from build123d import *

# Parameters (mm, degrees)
SKETCH_W               = 8.5
SKETCH_H               = 8.5
PAD_DEPTH              = 113.5
SKETCH001_W            = 10
SKETCH001_H            = 10
POCKET_DEPTH           = 2.5
LINEARPATTERN_COUNT    = 4
LINEARPATTERN_PITCH    = 20
SKETCH002_W            = 10
SKETCH002_H            = 10
POCKET001_DEPTH        = 2.5
LINEARPATTERN001_COUNT = 4
LINEARPATTERN001_PITCH = 20
FILLET_R               = 1
SKETCH003_R            = 1.25
POCKET002_DEPTH        = 6.001
LINEARPATTERN002_COUNT = 4
LINEARPATTERN002_PITCH = 20
SKETCH004_R            = 1.25
POCKET003_DEPTH        = 6.001
LINEARPATTERN003_COUNT = 4
LINEARPATTERN003_PITCH = 20


with BuildPart() as part:
    # Sketch → Pad (new body)
    with BuildSketch(Plane.XY):
        with Locations((4.25, 4.25)):
            Rectangle(SKETCH_W, SKETCH_H)
    extrude(amount=PAD_DEPTH)

    # Sketch001 → Pocket (cut)
    with BuildSketch(Plane.XZ):
        with Locations((4.410969, 21)):
            Rectangle(SKETCH001_W, SKETCH001_H)
    pocket = extrude(amount=-POCKET_DEPTH, mode=Mode.SUBTRACT)

    # LinearPattern: Pocket ×4
    with Locations(*[(0, 0, i * LINEARPATTERN_PITCH) for i in range(1, LINEARPATTERN_COUNT)]):
        add(pocket, mode=Mode.SUBTRACT)

    # Sketch002 → Pocket001 (cut)
    with BuildSketch(Plane(origin=(0, 0, 0), x_dir=(0, -1, 0), z_dir=(-1, 0, 0))):
        with Locations((-4.326825, 31)):
            Rectangle(SKETCH002_W, SKETCH002_H)
    pocket001 = extrude(amount=-POCKET001_DEPTH, mode=Mode.SUBTRACT)

    # LinearPattern001: Pocket001 ×4
    with Locations(*[(0, 0, i * LINEARPATTERN001_PITCH) for i in range(1, LINEARPATTERN001_COUNT)]):
        add(pocket001, mode=Mode.SUBTRACT)

    # Fillet
    fillet_edges = [part.edges().sort_by_distance(p)[0] for p in [
        (8.5, 8.5, 56.75),
    ]]
    fillet(fillet_edges, radius=FILLET_R)

    # Sketch003 → Pocket002 (cut, through all)
    with BuildSketch(Plane.XZ.offset(-2.5)):
        with Locations((5.25, 21)):
            Circle(SKETCH003_R)
    pocket002 = extrude(amount=-POCKET002_DEPTH, mode=Mode.SUBTRACT)

    # LinearPattern002: Pocket002 ×4
    with Locations(*[(0, 0, i * LINEARPATTERN002_PITCH) for i in range(1, LINEARPATTERN002_COUNT)]):
        add(pocket002, mode=Mode.SUBTRACT)

    # Sketch004 → Pocket003 (cut, through all)
    with BuildSketch(Plane(origin=(2.5, 0, 0), x_dir=(0, -1, 0), z_dir=(-1, 0, 0))):
        with Locations((-5.25, 31)):
            Circle(SKETCH004_R)
    pocket003 = extrude(amount=-POCKET003_DEPTH, mode=Mode.SUBTRACT)

    # LinearPattern003: Pocket003 ×4
    with Locations(*[(0, 0, i * LINEARPATTERN003_PITCH) for i in range(1, LINEARPATTERN003_COUNT)]):
        add(pocket003, mode=Mode.SUBTRACT)


solid = part.part
Build history of the part. All positions in model axes, mm. A direction names the side the tool comes from. Coordinates: 2 decimals unless noted, no trailing zeros. Write each loop counter-clockwise with the first axis right and the second up, starting at its lowest first coordinate (ties: lowest second). Pieces come first, ordered by that corner, then holes. Notation, with made-up numbers: (80.5, 18) -> (84.5, 18) arc R32 cw to (84.5, 52) -> close; hole circle Ø6 at (87.25, 72). An arc over 180 degrees is marked (long way). Use CSV: the item, a comma, the result in double quotes. Start each with the question number.
Q1. 3-axis set-ups, long thin cutter, end or side, ignore diameter. For faces 3 (the flat face through (2.5, 3, 91)), 4 (the cylindrical face through (5.46, 5.41, 52.24)), 5 (the flat face through (5, 1, 76)): which of +Z, -Z, +X, -X, +Y, -Y reach the whole face in a straight line?
Q2. Cut at B-B, the plane y = 5. State how many separate pieces and enclosed holes the cut face has, then the cut area to 3 significant figures.
Q3. Cut at C-C, the plane z = 44.5. List the corners of the cut face in (x, y), then the cut area to 3 significant figures.
Q4. Flat gauge pins, fed straight in: pin 1 Ø1.2 at (x, y) = (1.5, 5) entering from -Z; pin 2 Ø4 at (y, z) = (5.5, 29) entering from -X; pin 3 Ø2.5 at (x, z) = (4, 62) entering from -Y; pin 4 Ø1.5 at (x, z) = (5.25, 81) entering from +Y. Where does each tip first touch, or does it go through?
Q5. Cut at A-A, the plane z = 21. List the corners of the cut face in (x, y).
Q6. Pull direction Z, two halves, no side cores. Call faces 1 (the flat face through (4, 8.5, 56)), 2 (the flat face through (1, 6, 26)): released by +Z, released by -Z, zero draft, split by the parting line, or undercut.
Q7. Drill centre lines: probe 1 along Z at (x, y) = (5, 1); probe 2 along Z at (x, y) = (1, 7.25); probe 3 along Y at (x, z) = (6, 18). Where is each one in solid material? Low to high.
Checked values:
1,face 3,"-X, +Y, -Y"
1,face 4,"+X, -X"
1,face 5,"+X, -X, -Y"
2,separate pieces,"5"
2,enclosed holes,"4"
2,area,"786 mm²"
3,outline,"(0, 2.5) -> (8.5, 2.5) -> (8.5, 7.5) arc R1 ccw to (7.5, 8.5) -> (0, 8.5) -> close"
3,area,"50.8 mm²"
4,pin 1,"stops at z = 0"
4,pin 2,"stops at x = 2.5"
4,pin 3,"stops at y = 2.5"
4,pin 4,"passes through"
5,outline,"(0, 2.5) -> (4, 2.5) -> (4, 8.5) -> (0, 8.5) -> close; (6.5, 2.5) -> (8.5, 2.5) -> (8.5, 7.5) arc R1 ccw to (7.5, 8.5) -> (6.5, 8.5) -> close"
6,face 1,"zero draft"
6,face 2,"undercut"
7,probe 1,"z = 0 to 16, 26 to 36, 46 to 56, 66 to 76, 86 to 113.5"
7,probe 2,"z = 0 to 26, 36 to 46, 56 to 66, 76 to 86, 96 to 113.5"
7,probe 3,"y = 2.5 to 8.5"
